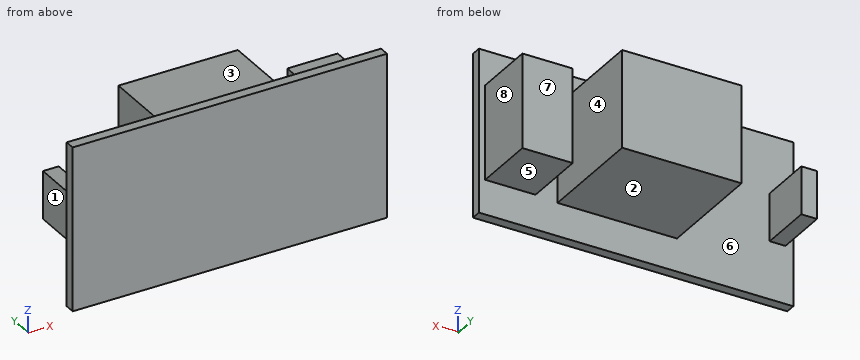
```python
from build123d import *

# Parameters (mm, degrees)
SKETCH1_W            = 50
SKETCH1_H            = 26
BOARD_DEPTH          = 1.6
RELAY_START          = 1.6
SKETCH2_W            = 19
SKETCH2_H            = 15.5
RELAY_DEPTH          = 17.4
TERMINAL_BLOCK_START = 1.6
SKETCH3_W            = 8
SKETCH3_H            = 15
TERMINAL_BLOCK_DEPTH = 10
HEADER_START         = 1.6
SKETCH4_W            = 2.5
SKETCH4_H            = 7.6
HEADER_DEPTH         = 8.5


with BuildPart() as part:
    # Sketch1 → Board (new body)
    with BuildSketch(Plane(origin=(0, 0, 0), x_dir=(1, 0, 0), z_dir=(0, 1, 0))):
        Rectangle(SKETCH1_W, SKETCH1_H)
    extrude(amount=BOARD_DEPTH)

    # Sketch2 → Relay (add)
    with BuildSketch(Plane(origin=(0, 0, 0), x_dir=(1, 0, 0), z_dir=(0, 1, 0)).offset(RELAY_START)):
        with Locations((3, 0)):
            Rectangle(SKETCH2_W, SKETCH2_H)
    extrude(amount=RELAY_DEPTH)

    # Sketch3 → Terminal_Block (add)
    with BuildSketch(Plane(origin=(0, 0, 0), x_dir=(1, 0, 0), z_dir=(0, 1, 0)).offset(TERMINAL_BLOCK_START)):
        with Locations((20, 0)):
            Rectangle(SKETCH3_W, SKETCH3_H)
    extrude(amount=TERMINAL_BLOCK_DEPTH)

    # Sketch4 → Header (add)
    with BuildSketch(Plane(origin=(0, 0, 0), x_dir=(1, 0, 0), z_dir=(0, 1, 0)).offset(HEADER_START)):
        with Locations((-22.5, 0)):
            Rectangle(SKETCH4_W, SKETCH4_H)
    extrude(amount=HEADER_DEPTH)


solid = part.part
```
Geometry: final body of the model. Coordinates: model frame, mm. Face numbers are marked on the shaded views. A direction names the side the tool comes from. Coordinates: 2 decimals unless noted, no trailing zeros. Order: outer loops, then holes, each group sorted by start corner. A loop starts at its lowest first (then second) coordinate and runs counter-clockwise, first axis right, second up. Notation, with made-up numbers: M -13.75,-10 L -5.75,-10 A16 cw -5.75,7 Z; hole C 89.25,-26.5 d9. An arc over 180 degrees is marked long. Answer in a Markdown table with one row per item. Add a question column.
Q1. Section query D-D on y = 14.25. Return the cut outline in (x, z), and give its area (4 significant figures).
Q2. Section query C-C on z = 5.5. Return the cut outline in (x, y).
Q3. Mould query, pull axis X, two halves, no side actions, for the marked faces 6, 7 and 8. Classes: released by +X, released by -X, zero draft, split by the parting line, or undercut.
Q4. Contact query for flat-ended pins moving along their axis: P1, Ø2, axis at x = -23, y = 6.5, coming from the +Z side; P2, Ø5, axis at x = 12.5, y = 7, coming from the +Z side; P3, Ø3, axis at x = -22, y = 6, coming from the -Z side; P4, Ø2, axis at x = 17, z = 9.5, coming from the -Y side. Output: stop coordinate, or through.
Q5. Section query B-B on x = 19. Return the cut outline in (y, z).
Q6. Reachability of the marked faces 1, 2, 3, 4 and 5 from +Z, -Z, +X, -X, +Y, -Y: full face, straight path, thin tool, end or side. Return the list, or none.
Q7. Section query A-A on y = 6. Return the cut outline in (x, z), and give its area (4 significant figures).
Q8. Line query: L1, parallel to X at y = 7.5, z = -2.75; L2, parallel to X at y = 1.75, z = 4; L3, parallel to X at y = 13, z = 1.25. Output: solid intervals per line, ascending.
Completed:
| question | item | result |
|---|---|---|
| 1 | outline | M -6.5,-7.75 L 12.5,-7.75 L 12.5,7.75 L -6.5,7.75 Z |
| 1 | area | 294.5 mm2 |
| 2 | outline | M -25,0 L 25,0 L 25,1.6 L 24,1.6 L 24,11.6 L 16,11.6 L 16,1.6 L 12.5,1.6 L 12.5,19 L -6.5,19 L -6.5,1.6 L -25,1.6 Z |
| 3 | face 6 | undercut |
| 3 | face 7 | zero draft |
| 3 | face 8 | released by +X |
| 4 | P1 | stops at z = 3.8 |
| 4 | P2 | stops at z = 7.75 |
| 4 | P3 | stops at z = -3.8 |
| 4 | P4 | stops at y = 0 |
| 5 | outline | M 0,-13 L 1.6,-13 L 1.6,-7.5 L 11.6,-7.5 L 11.6,7.5 L 1.6,7.5 L 1.6,13 L 0,13 Z |
| 6 | face 1 | +Z, -Z, -X, +Y |
| 6 | face 2 | -Z, +X, -X, +Y |
| 6 | face 3 | +Z, +X, -X, +Y |
| 6 | face 4 | +Z, -Z, +Y |
| 6 | face 5 | -Z, +X, +Y |
| 7 | outline | M -23.75,-3.8 L -21.25,-3.8 L -21.25,3.8 L -23.75,3.8 Z; M -6.5,-7.75 L 12.5,-7.75 L 12.5,7.75 L -6.5,7.75 Z; M 16,-7.5 L 24,-7.5 L 24,7.5 L 16,7.5 Z |
| 7 | area | 433.5 mm2 |
| 8 | L1 | x = -23.75 to -21.25, -6.5 to 12.5, 16 to 24 |
| 8 | L2 | x = -6.5 to 12.5, 16 to 24 |
| 8 | L3 | x = -6.5 to 12.5 |
